Geometry check sheet. Reference: the model listing, model coordinates, mm. A direction names the side the tool comes from. Round coordinates to 2 decimals unless told otherwise and drop trailing zeros. Order: outer loops, then holes, each group sorted by start corner. A loop starts at its lowest first (then second) coordinate and runs counter-clockwise, first axis right, second up. Notation, with made-up numbers: (25, -29) -> (59, -29) arc R19 cw to (59, -1) -> close; hole circle Ø8 at (41.25, -37). An arc over 180 degrees is marked (long way). Use a Markdown table: item, result. Add a question column.
Item 1: Material ranges on probe 1 along Z at (x, y) = (25.4, 13.5); probe 2 along Z at (x, y) = (25.4, 22.25); probe 3 along Z at (x, y) = (48.5, 3), recorded low to high. Write a range as [from, to].
Item 2: Sectioned sample at A-A, the plane x = 25.4. Record the cut outline in (y, z), and give its area (3 significant figures).
Item 3: Mould release check, pull along Z, two halves, no side actions. Record for faces 1 (the cylindrical face through (23.747, 16.05, 63.392)), 2 (the flat face through (25, 16, 0)), 3 (the flat face through (25, 0, 3)): pulls with the +Z half, pulls with the -Z half, needs draft (parallel to the pull), parting line crosses it, or undercut.
Item 4: Sectioned sample at D-D, the plane y = 21. Record the cut outline in (x, z).
Item 5: Sectioned sample at B-B, the plane y = 15.5. Record the cut outline in (x, z).
Item 6: Gauge pin test, flat ends, axial feed: pin 1 Ø8 at (x, z) = (23, 50.5) entering from +Y; pin 2 Ø6.5 at (y, z) = (24.5, 41.5) entering from -X; pin 3 Ø10 at (y, z) = (22.5, 17) entering from +X; pin 4 Ø1 at (x, z) = (33.5, 7.5) entering from -Y. Record the tip position at first contact, or that the pin passes through.
Item 7: Set-up check for faces 4 (the flat face through (25, 31.75, 25)), 5 (the flat face through (25, 9, 6.35)), 6 (the flat face through (12.7, 25, 35)), 7 (the flat face through (38.1, 25, 35)), 8 (the flat face through (28, 6.35, 57)): record each of +Z, -Z, +X, -X, +Y, -Y from which the full face is reachable in a straight line by a thin tool's end or side.
Item 8: Sectioned sample at C-C, the plane z = 5. Record the cut outline in (x, y) (3 decimals).
from build123d import *
from build123d import SkipClean  # not in build123d's __all__

# Parameters (mm, degrees)
F0_W     = 50.8
F0_H     = 6.35
F1_DEPTH = 31.75
F3_DEPTH = 19.05
F4_DEPTH = 6.35
F6_DEPTH = 6.351


with BuildPart() as f1:
    # F0 (on Front) → F1 (new body)
    with BuildSketch(Plane.XZ):
        with Locations((25.4, 3.175)):
            Rectangle(F0_W, F0_H)
        with BuildLine():
            ThreePointArc((12.7, 19.05), (8.9802561211, 10.0697438789), (0, 6.35))
            Line((0, 6.35), (50.8, 6.35))
            ThreePointArc((50.8, 6.35), (41.8197438789, 10.0697438789), (38.1, 19.05))
            Line((38.1, 19.05), (38.1, 50.8))
            ThreePointArc((38.1, 50.8), (25.4, 38.1), (12.7, 50.8))
            Line((12.7, 50.8), (12.7, 19.05))
        make_face()
        with BuildLine():
            Line((19.05, 50.8), (12.7, 50.8))
            ThreePointArc((12.7, 50.8), (25.4, 38.1), (38.1, 50.8))
            Line((38.1, 50.8), (31.75, 50.8))
            ThreePointArc((31.75, 50.8), (25.4, 44.45), (19.05, 50.8))
        make_face()
        with BuildLine():
            ThreePointArc((38.1, 50.8), (25.4, 63.5), (12.7, 50.8))
            Line((12.7, 50.8), (19.05, 50.8))
            ThreePointArc((19.05, 50.8), (25.4, 57.15), (31.75, 50.8))
            Line((31.75, 50.8), (38.1, 50.8))
        make_face()
    extrude(amount=-F1_DEPTH)

    # F2 (on face) → F3 (cut)
    with BuildSketch(Plane.XZ):
        with BuildLine():
            ThreePointArc((12.7, 19.05), (8.9802561211, 10.0697438789), (0, 6.35))
            Line((0, 6.35), (50.8, 6.35))
            ThreePointArc((50.8, 6.35), (41.8197438789, 10.0697438789), (38.1, 19.05))
            Line((38.1, 19.05), (38.1, 50.8))
            ThreePointArc((38.1, 50.8), (25.4, 38.1), (12.7, 50.8))
            Line((12.7, 50.8), (12.7, 19.05))
        make_face()
    with SkipClean():  # cleaning this boolean's faces spoils the solid; the shape is the same uncleaned
        extrude(amount=-F3_DEPTH, mode=Mode.SUBTRACT)

    # F4 (cut): a face of the model
    f4_faces = [f1.faces().sort_by_distance(p)[0] for p in [
        (25.4, 0, 63.1407897552),
    ]]
    extrude(f4_faces, amount=-F4_DEPTH, mode=Mode.SUBTRACT)

    # F5 (on face) → F6 (cut, through all)
    with BuildSketch(Plane.XY.offset(6.35)):
        with BuildLine():
            ThreePointArc((12.7, 9.525), (11.2473638622, 12.1922247236), (8.2186848968, 12.4188151032))
            ThreePointArc((8.2186848968, 12.4188151032), (10.3079286634, 11.3156118148), (11.849261314, 9.525))
            Line((11.849261314, 9.525), (12.7, 9.525))
        make_face()
        with BuildLine():
            ThreePointArc((11.849261314, 9.525), (10.3079286634, 11.3156118148), (8.2186848968, 12.4188151032))
            ThreePointArc((8.2186848968, 12.4188151032), (6.8577752764, 11.2473638622), (6.35, 9.525))
            Line((6.35, 9.525), (11.849261314, 9.525))
        make_face()
        with BuildLine():
            ThreePointArc((6.35, 9.525), (8.8568824776, 6.4210921444), (12.4188151032, 8.2186848968))
            ThreePointArc((12.4188151032, 8.2186848968), (12.1708000125, 8.8878706063), (11.849261314, 9.525))
            Line((11.849261314, 9.525), (6.35, 9.525))
        make_face()
        with BuildLine():
            ThreePointArc((11.849261314, 9.525), (12.1708000125, 8.8878706063), (12.4188151032, 8.2186848968))
            ThreePointArc((12.4188151032, 8.2186848968), (12.6289078556, 8.8568824776), (12.7, 9.525))
            Line((12.7, 9.525), (11.849261314, 9.525))
        make_face()
        with BuildLine():
            ThreePointArc((38.950738686, 9.525), (40.4920713366, 11.3156118148), (42.5813151032, 12.4188151032))
            ThreePointArc((42.5813151032, 12.4188151032), (39.5526361378, 12.1922247236), (38.1, 9.525))
            Line((38.1, 9.525), (38.950738686, 9.525))
        make_face()
        with BuildLine():
            ThreePointArc((44.45, 9.525), (43.9422247236, 11.2473638622), (42.5813151032, 12.4188151032))
            ThreePointArc((42.5813151032, 12.4188151032), (40.4920713366, 11.3156118148), (38.950738686, 9.525))
            Line((38.950738686, 9.525), (44.45, 9.525))
        make_face()
        with BuildLine():
            ThreePointArc((38.950738686, 9.525), (38.6291999875, 8.8878706063), (38.3811848968, 8.2186848968))
            ThreePointArc((38.3811848968, 8.2186848968), (41.9431175224, 6.4210921444), (44.45, 9.525))
            Line((44.45, 9.525), (38.950738686, 9.525))
        make_face()
        with BuildLine():
            ThreePointArc((38.1, 9.525), (38.1710921444, 8.8568824776), (38.3811848968, 8.2186848968))
            ThreePointArc((38.3811848968, 8.2186848968), (38.6291999875, 8.8878706063), (38.950738686, 9.525))
            Line((38.950738686, 9.525), (38.1, 9.525))
        make_face()
        with BuildLine():
            Line((44.45, 0), (50.8, 0))
            Line((50.8, 0), (50.8, 6.35))
            ThreePointArc((50.8, 6.35), (48.9401280605, 1.8598719395), (44.45, 0))
        make_face()
        with BuildLine():
            Line((0, 0), (6.35, 0))
            ThreePointArc((6.35, 0), (1.8598719395, 1.8598719395), (0, 6.35))
            Line((0, 6.35), (0, 0))
        make_face()
    extrude(amount=-F6_DEPTH, mode=Mode.SUBTRACT)


solid = f1.part
Found:
| question | item | result |
|---|---|---|
| 1 | probe 1 | z = [0, 6.35], [38.1, 44.45], [57.15, 63.5] |
| 1 | probe 2 | z = [0, 44.45], [57.15, 63.5] |
| 1 | probe 3 | z = [0, 6.35] |
| 2 | outline | (0, 0) -> (31.75, 0) -> (31.75, 44.45) -> (6.35, 44.45) -> (6.35, 38.1) -> (19.05, 38.1) -> (19.05, 6.35) -> (0, 6.35) -> close; (6.35, 57.15) -> (31.75, 57.15) -> (31.75, 63.5) -> (6.35, 63.5) -> close |
| 2 | area | 927 mm2 |
| 3 | face 1 | undercut |
| 3 | face 2 | pulls with the -Z half |
| 3 | face 3 | needs draft |
| 4 | outline | (0, 0) -> (50.8, 0) -> (50.8, 6.35) arc R12.7 cw to (38.1, 19.05) -> (38.1, 50.8) arc R12.7 ccw to (12.7, 50.8) -> (12.7, 19.05) arc R12.7 cw to (0, 6.35) -> close; hole circle Ø12.7 at (25.4, 50.8) |
| 5 | outline | (0, 0) -> (50.8, 0) -> (50.8, 6.35) -> (0, 6.35) -> close; circle Ø25.4 at (25.4, 50.8); hole circle Ø12.7 at (25.4, 50.8) |
| 6 | pin 1 | stops at y = 31.75 |
| 6 | pin 2 | stops at x = 12.7 |
| 6 | pin 3 | stops at x = 40.24 |
| 6 | pin 4 | stops at y = 19.05 |
| 7 | face 4 | +Z, -Z, +X, -X, +Y |
| 7 | face 5 | +X, -X, -Y |
| 7 | face 6 | +Z, -X, +Y, -Y |
| 7 | face 7 | +Z, +X, +Y, -Y |
| 7 | face 8 | +Z, +X, -X, -Y |
| 8 | outline | (0, 6.35) arc R6.35 ccw to (6.35, 0) -> (44.45, 0) arc R6.35 ccw to (50.8, 6.35) -> (50.8, 31.75) -> (0, 31.75) -> close; hole circle Ø6.35 at (9.525, 9.525); hole circle Ø6.35 at (41.275, 9.525) |
